```python
from build123d import *

# Parameters (mm, degrees)
BOSS_EXTRU_1_DEPTH       = 40
D_GAGEMENT_START         = 54.723222932
D_GAGEMENT_M22_OUTLINE_R = 1.2
D_GAGEMENT_M22_DEPTH     = 5
ENL_V_MAT_EXTRU_3_REACH  = 166.408
ESQUISSE12_W             = 11.5
ESQUISSE12_H             = 18.5
CONG_2_R                 = 1
ENL_V_MAT_EXTRU_4_REACH  = 205.438


# Read off the part's stored shape, not the designer's step: Dégagement M22
with BuildPart() as part:
    # Esquisse1 → Boss.-Extru.1 (new body)
    with BuildSketch(Plane.XY):
        Polygon((0, 0), (10, 0), (10, 160), (5.320888862, 160), (-8.982342629, 199.297805548), (-13.680805733, 197.587704831), (0, 160), align=None)
    extrude(amount=BOSS_EXTRU_1_DEPTH)

    # Dégagement M22 outline → Dégagement M22 (cut)
    with BuildSketch(Plane(origin=(0, 0, 0), x_dir=(-0.3420201433256691, 0.9396926207859082, 0), z_dir=(0.9396926207859083, 0.3420201433256691, 0)).offset(D_GAGEMENT_START)):
        with Locations((162.600819326, 30.25)):
            Circle(D_GAGEMENT_M22_OUTLINE_R)
        with Locations((175.100819326, 9.75)):
            Circle(D_GAGEMENT_M22_OUTLINE_R)
        with Locations((175.100819326, 30.25)):
            Circle(D_GAGEMENT_M22_OUTLINE_R)
        with Locations((162.600819326, 9.75)):
            Circle(D_GAGEMENT_M22_OUTLINE_R)
    extrude(amount=D_GAGEMENT_M22_DEPTH, mode=Mode.SUBTRACT)

    # Esquisse12 → Enlèv. mat.-Extru.3 (cut, up to next)
    with BuildSketch(Plane(origin=(39.231681983, 52.211839625, 50.949763499), x_dir=(0, 0, 1), z_dir=(-0.9396926207859084, -0.3420201433256691, 0)), mode=Mode.PRIVATE) as enl_v_mat_extru_3_sk1:
        with Locations((-30.949763499, 130.455764407)):
            Rectangle(ESQUISSE12_W, ESQUISSE12_H)
    enl_v_mat_extru_3_tool1 = extrude(enl_v_mat_extru_3_sk1.sketch, amount=-ENL_V_MAT_EXTRU_3_REACH, mode=Mode.PRIVATE) & part.part
    add(enl_v_mat_extru_3_tool1.solids().sort_by_distance((-5.386817, 174.800159, 20))[0], mode=Mode.SUBTRACT)

    # Congé2
    cong_2_edges = [part.edges().sort_by_distance(p)[0] for p in [
        (0, 80, 0),
        (0, 160, 20),
        (-13.680805733, 197.587704831, 20),
        (-8.982342629, 199.297805548, 20),
        (10, 80, 40),
        (5.320888862, 160, 20),
        (10, 160, 20),
        (10, 0, 20),
        (0, 0, 20),
        (7.660444431, 160, 40),
        (-1.830726883, 179.648902774, 40),
        (-11.331574181, 198.44275519, 40),
        (-6.840402867, 178.793852416, 40),
        (0, 80, 40),
        (-6.840402867, 178.793852416, 0),
        (-11.331574181, 198.44275519, 0),
        (-1.830726883, 179.648902774, 0),
        (7.660444431, 160, 0),
        (5, 0, 40),
        (10, 80, 0),
        (5, 0, 0),
    ]]
    fillet(cong_2_edges, radius=CONG_2_R)

    # Esquisse13 → Enlèv. mat.-Extru.4 (cut, up to next)
    with BuildSketch(Plane.ZY, mode=Mode.PRIVATE) as enl_v_mat_extru_4_sk1:
        with BuildLine():
            Line((8.55, 7.5), (8.55, 127.5))
            ThreePointArc((8.55, 127.5), (10, 128.95), (11.45, 127.5))
            Line((11.45, 127.5), (11.45, 7.5))
            ThreePointArc((11.45, 7.5), (10, 6.05), (8.55, 7.5))
        make_face()
    enl_v_mat_extru_4_tool1 = extrude(enl_v_mat_extru_4_sk1.sketch, amount=-ENL_V_MAT_EXTRU_4_REACH, mode=Mode.PRIVATE) & part.part
    # Esquisse13 → Enlèv. mat.-Extru.4 (cut, up to next)
    with BuildSketch(Plane.ZY, mode=Mode.PRIVATE) as enl_v_mat_extru_4_sk2:
        with BuildLine():
            Line((28.55, 7.5), (28.55, 127.5))
            ThreePointArc((28.55, 127.5), (30, 128.95), (31.45, 127.5))
            Line((31.45, 127.5), (31.45, 7.5))
            ThreePointArc((31.45, 7.5), (30, 6.05), (28.55, 7.5))
        make_face()
    enl_v_mat_extru_4_tool2 = extrude(enl_v_mat_extru_4_sk2.sketch, amount=-ENL_V_MAT_EXTRU_4_REACH, mode=Mode.PRIVATE) & part.part
    add(enl_v_mat_extru_4_tool1.solids().sort_by_distance((0, 67.5, 10))[0], mode=Mode.SUBTRACT)
    add(enl_v_mat_extru_4_tool2.solids().sort_by_distance((0, 67.5, 30))[0], mode=Mode.SUBTRACT)


solid = part.part
```
Source: CAD feature listing. Evaluate the final solid. Frame: model axes, mm. A direction names the side the tool comes from. Give positions to 0.01 mm unless a question says otherwise; leave off trailing zeros. Order: outer loops, then holes, each group sorted by start corner. A loop starts at its lowest first (then second) coordinate and runs counter-clockwise, first axis right, second up.
(1) Access query for faces 4 (the face through (-2.158, 179.669, 0.285)), 5 (the face through (0.09, 166.95, 19.92)), 6 (the face through (-6.234, 184.335, 19.92)), 7 (the face through (5, 67, 28.55)). Directions: +Z, -Z, +X, -X, +Y, -Y. A direction counts if a zero-diameter tool reaches every point of the face in a straight line with its end or side. Return the directions, or none.
(2) Section query D-D (x = -6.25). State how many separate pieces and enclosed holes the cut face has, plus the area to 3 significant figures.
(3) Contact query for flat-ended pins moving along their axis: P1, Ø6, axis at y = 123.5, z = 34, coming from the -X side; P2, Ø6, axis at y = 169, z = 27, coming from the -X side; P3, Ø1.5, axis at x = 7, z = 27.5, coming from the +Y side; P4, Ø3.5, axis at x = -2, y = 180, coming from the +Z side. Output: stop coordinate, or through.
(4) Section query B-B (z = 6). Return the cut outline in (x, y), plus the area to 3 significant figures.
(5) Material intervals for line 1 along Z through (x, y) = (6.5, 111); line 2 along Z through (x, y) = (-5.5, 177.5); line 3 along X through (y, z) = (30.5, 3), sorted ascending.
(6) Section query A-A (y = 75.5). Return the cut outline in (x, z), plus the area to 3 significant figures.
(7) Pull-direction query (X, two-part tool) for faces 1 (the face through (10, 79, 20)), 2 (the face through (-6.54, 185.176, 30.61)), 3 (the face through (5, 67, 8.55)); classes: +X half, -X half, draft (parallel to the pull), parting line (faces both ways), or undercut.
(8) Section query C-C (y = 152). Return the cut outline in (x, z).
Outcome:
1. face 4: -Z, +X, +Y
1. face 5: -X, +Y
1. face 6: +X, -Y
1. face 7: +X, -X
2. separate pieces: 1
2. enclosed holes: 2
2. area: 490 mm2
3. P1: stops at x = 0
3. P2: stops at x = -4.37
3. P3: stops at y = 160
3. P4: stops at z = 40
4. outline: (-13.34, 196.65) - (-0.06, 160.17) arc R1 cw to (0, 159.82) - (0, 1) arc R1 ccw to (1, 0) - (9, 0) arc R1 ccw to (10, 1) - (10, 159) arc R1 ccw to (9, 160) - (6.02, 160) arc R1 cw to (5.08, 160.66) - (-8.64, 198.36) arc R1 ccw to (-9.92, 198.96) - (-12.74, 197.93) arc R1 ccw to start
4. area: 1,800 mm2
5. line 1: z = 0 to 8.55, 11.45 to 28.55, 31.45 to 40
5. line 2: z = 0.02 to 14.25, 25.75 to 39.98
5. line 3: x = 0 to 10
6. outline: (0, 1) arc R1 ccw to (1, 0) - (9, 0) arc R1 ccw to (10, 1) - (10, 8.55) - (0, 8.55) - close; (0, 11.45) - (10, 11.45) - (10, 28.55) - (0, 28.55) - close; (0, 31.45) - (10, 31.45) - (10, 39) arc R1 ccw to (9, 40) - (1, 40) arc R1 ccw to (0, 39) - close
6. area: 341 mm2
7. face 1: +X half
7. face 2: undercut
7. face 3: draft
8. outline: (0, 1) arc R1 ccw to (1, 0) - (9, 0) arc R1 ccw to (10, 1) - (10, 39) arc R1 ccw to (9, 40) - (1, 40) arc R1 ccw to (0, 39) - close
